Build history of the part. All positions in model axes, mm. Give positions to 0.01 mm unless a question says otherwise; leave off trailing zeros. Write each loop counter-clockwise with the first axis right and the second up, starting at its lowest first coordinate (ties: lowest second). Pieces come first, ordered by that corner, then holes. Notation, with made-up numbers: (32.25, 18) -> (61.25, 18) arc R26 ccw to (61.25, 40) -> close; hole circle Ø8 at (78.5, 16.5). An arc over 180 degrees is marked (long way). Write item = value, one per line. Start each with the question number.
Q1. Wall check: line 1 (Y direction, x = 0, z = 0.6); line 2 (X direction, y = 4.5, z = 1.4); line 3 (Y direction, x = -15, z = 0.9). Give the ranges that are in metal, low to high.
Q2. Saw through at B-B, the plane y = -18.5. List the corners of the cut face in (x, z).
Q3. Saw through at C-C, the plane y = 2.5. List the corners of the cut face in (x, z), then the cut area to 3 significant figures.
Q4. Drop flat-ended pins along their axis: P1, Ø1.9, axis at x = 15, y = 16.5, coming from the -Z side; P2, Ø10, axis at x = 13, y = 11.5, coming from the -Z side; P3, Ø1, axis at y = 6.5, z = 1.5, coming from the +X side. Give the stop position or say it passes through.
Q5. Saw through at D-D, the plane z = 1.05. Give the number of separate pieces and of enclosed holes in the cut face, then the cut area to 3 significant figures.
Q6. Saw through at A-A, the plane x = 0. List the corners of the cut face in (y, z).
Autodesk Inventor part; units mm, degrees
ref_plane "YZ Plane" through (0, 0, 0) normal (1, 0, 0) x (0, 1, 0)
ref_plane "XZ Plane" through (0, 0, 0) normal (0, 1, 0) x (-1, 0, 0)
ref_plane "XY Plane" through (0, 0, 0) normal (0, 0, 1) x (1, 0, 0)
sketch "スケッチ1" plane through (0, 0, 0) normal (0, 0, 1) x (1, 0, 0)
  circle A0 centre (0, 0) radius 11
  line L0 (-10, 22) -> (10, 22)
  line L1 (17.75, -44.5) -> (-17.75, -44.5)
  line L2 (-15, 16.5) -> (15, 16.5) construction
  line L3 (15, 16.5) -> (15, -42) construction
  line L4 (15, -42) -> (-15, -42) construction
  line L5 (-15, -42) -> (-15, 16.5) construction
  circle A1 centre (-15, 16.5) radius 1.55
  circle A2 centre (15, 16.5) radius 1.55
  circle A3 centre (-15, -42) radius 1.55
  circle A4 centre (15, -42) radius 1.55
  line L6 (-17.75, -44.5) -> (-20, -44.5)
  line L7 (-20, -44.5) -> (-20, 17.12)
  line L8 (-10, 22) -> (-20, 17.12)
  line L9 (0, 22) -> (0, -44.5) construction
  line L10 (-20, -23) -> (-22, -23)
  line L11 (-22, -23) -> (-22, -13)
  line L12 (-22, -13) -> (-20, -13)
  line L13 (17.75, -44.5) -> (20, -44.5)
  line L14 (20, -44.5) -> (20, 17.12)
  line L15 (10, 22) -> (20, 17.12)
  line L16 (20, -23) -> (22, -23)
  line L17 (22, -23) -> (22, -13)
  line L18 (22, -13) -> (20, -13)
  line L19 (13.5, -1) -> (-13.5, -1) construction
  line L20 (-13.5, -1) -> (-13.5, -28) construction
  line L21 (-13.5, -28) -> (13.5, -28) construction
  line L22 (13.5, -28) -> (13.5, -1) construction
  circle A5 centre (-13.5, -1) radius 1.35
  circle A6 centre (-13.5, -28) radius 1.35
  circle A7 centre (13.5, -1) radius 1.35
  circle A8 centre (13.5, -28) radius 1.35
  line L23 (10.01, -42) -> (-10.01, -42)
  line L24 (-10.01, -42) -> (-10.01, -39.48)
  line L25 (-10.01, -39.48) -> (10.01, -39.48)
  line L26 (10.01, -39.48) -> (10.01, -42)
  circle A9 centre (-8.96, -39.48) radius 1.05
  circle A10 centre (-8.96, -42) radius 1.05
  circle A11 centre (8.96, -42) radius 1.05
  circle A12 centre (8.96, -39.48) radius 1.05
  line L27 (-10.1, 19.01) -> (10.1, 19.01)
  line L28 (10.1, 19.01) -> (10.1, 16.49)
  line L29 (10.1, 16.49) -> (-10.1, 16.49)
  line L30 (-10.1, 16.49) -> (-10.1, 19.01)
  circle A13 centre (-9.05, 19.01) radius 1.05
  circle A14 centre (-9.05, 16.49) radius 1.05
  circle A15 centre (9.05, 16.49) radius 1.05
  circle A16 centre (9.05, 19.01) radius 1.05
  arc A17 (-20, -25.1) -> (-20, -23) centre (-20, -24.05) ccw
  arc A18 (-20, -13) -> (-20, -10.9) centre (-20, -11.95) ccw
  arc A19 (20, -23) -> (20, -25.1) centre (20, -24.05) ccw
  arc A20 (20, -10.9) -> (20, -13) centre (20, -11.95) ccw
  point P0 (7.91, -42)
  point P1 (-7.91, -42)
  point P2 (-7.91, -39.48)
  point P3 (7.91, -39.48)
  point P4 (8, 16.49)
  point P5 (-8, 16.49)
  point P6 (-10.1, 19.01)
  point P7 (-8, 19.01)
  point P8 (8, 19.01)
  point P9 (0, -39.48)
  point P10 (0, 16.49)
  point P11 (0, 19.01)
  point P12 (20, -25.1)
  dimension "d111" = 2.1
  dimension "d140" = 2.1
  dimension "d141" = 2.1
  dimension "d147" = 2.1
  dimension "d0" = 22
  dimension "d1" = 20
  dimension "d3" = 35.5
  dimension "d6" = 44.5
  dimension "d12" = 66.5
  dimension "d21" = 58.5
  dimension "d23" = 5.5
  dimension "d25" = 3.1
  dimension "d26" = 3.1
  dimension "d27" = 3.1
  dimension "d28" = 3.1
  dimension "d38" = 2
  dimension "d39" = 10
  dimension "d42" = 15
  dimension "d43" = 30
  dimension "d44" = 35
  dimension "d45" = 15
  dimension "d62" = 27
  dimension "d63" = 27
  dimension "d64" = 13.5
  dimension "d65" = 1
  dimension "d66" = 2.7
  dimension "d67" = 2.7
  dimension "d68" = 2.7
  dimension "d69" = 2.7
  dimension "d104" = 20.02
  dimension "d105" = 2.52
  dimension "d109" = 2.1
  dimension "d110" = 2.1
  dimension "d112" = 2.1
  dimension "d129" = 16.5
  dimension "d131" = 39.48
  dimension "d133" = 2.52
  dimension "d134" = 20.2
  dimension "d136" = 5.51
  dimension "d139" = 2.1
  dimension "d149" = 40
  dimension "d150" = 2.75
  dimension "d151" = 1.05
  dimension "d152" = 1.05
extrude "押し出し1" add sketch "スケッチ1" along normal blind 2 contours L0 L15 L14 A20 A19 L13 L1 L6 L7 A17 A18 L8 | L7 L10 L11 L12 | L18 L17 L16 L14
sketch "スケッチ2" plane through (0, 0, 2) normal (0, 0, 1) x (1, 0, 0)
  circle A0 centre (-13.5, -28) radius 1.35
  circle A1 centre (13.5, -28) radius 1.35
  circle A2 centre (-13.5, -1) radius 1.35
  circle A3 centre (13.5, -1) radius 1.35
  circle A4 centre (0, 0) radius 13 construction
  line L0 (20, -44.5) -> (20, 17.12)
  line L1 (-20, 17.12) -> (-20, -44.5)
  line L2 (10, 22) -> (-10, 22)
  line L3 (0, 22) -> (0, -44.5) construction
  line L4 (-20, -44.5) -> (20, -44.5)
  circle A5 centre (-13.5, -1) radius 2.6 construction
  circle A6 centre (13.5, -1) radius 2.6 construction
  circle A7 centre (-13.5, -28) radius 2.6 construction
  circle A8 centre (13.5, -28) radius 2.6 construction
  arc A9 (-3.8182, 12.4266) -> (-12.8912, 1.6787) centre (0, 0) ccw
  arc A10 (12.8912, 1.6787) -> (3.8182, 12.4266) centre (0, 0) ccw
  arc A11 (-12.4916, -3.6) -> (12.4916, -3.6) centre (0, 0) ccw
  arc A12 (-10.9, -28) -> (-13.5, -25.4) centre (-13.5, -28) ccw
  arc A13 (13.5, -25.4) -> (10.9, -28) centre (13.5, -28) ccw
  line L5 (-10.9, -28) -> (10.9, -28)
  line L6 (-13.4907, -30.6) -> (13.5093, -30.6)
  arc A14 (-7.91, -39.48) -> (-10.01, -39.48) centre (-8.96, -39.48) ccw
  circle A15 centre (-8.96, -39.48) radius 2.45 construction
  arc A16 (10.01, -39.48) -> (7.91, -39.48) centre (8.96, -39.48) ccw
  circle A17 centre (8.96, -39.48) radius 2.45 construction
  line L7 (-13.4907, -30.6) -> (-13.4907, -37.03)
  line L8 (-13.4907, -37.03) -> (13.5093, -37.03)
  line L9 (13.5093, -37.03) -> (13.5093, -30.6)
  line L10 (-17.5, 12.5022) -> (-3.8182, 12.4266)
  line L11 (-17.5, 12.5022) -> (-17.5, 1.6787)
  line L12 (-17.5, 1.6787) -> (-12.8912, 1.6787)
  arc A18 (12.8912, 1.6787) -> (3.8182, 12.4266) centre (0, 0) ccw
  line L13 (17.5, 12.5022) -> (3.8182, 12.4266)
  line L14 (17.5, 12.5022) -> (17.5, 1.6787)
  line L15 (17.5, 1.6787) -> (12.8912, 1.6787)
  line L16 (-17.48, -3.6) -> (-12.4916, -3.6)
  line L17 (-17.48, -3.6) -> (-17.48, -25.4)
  line L18 (-17.48, -25.4) -> (-13.5, -25.4)
  line L19 (17.5, -3.6) -> (12.4916, -3.6)
  line L20 (17.5, -3.6) -> (17.5, -25.4)
  line L21 (17.5, -25.4) -> (13.5, -25.4)
  dimension "d76" = 26
  dimension "d82" = 5.2
  dimension "d83" = 5.2
  dimension "d84" = 5.2
  dimension "d85" = 5.2
  dimension "d88" = 23.8182
  dimension "d89" = 32.8912
  dimension "d92" = 21.8
  dimension "d94" = 13
  dimension "d115" = 4.9
  dimension "d116" = 4.9
  dimension "d117" = 6.5093
  dimension "d118" = 7.47
  dimension "d123" = 10.8236
  dimension "d124" = 2.5
  dimension "d125" = 21.8
  dimension "d126" = 34.98
  dimension "d127" = 2.5
extrude "押し出し2" cut sketch "スケッチ2" against normal blind 2 contours A9 L12 L11 L10 | A10 L13 L14 L15 | A11 L19 L20 L21 A13 L5 A12 L18 L17 L16 | L6 L9 L8 L7
fillet "フィレット2" radius 2 20 edges at (-17.5, 12.5022, 1) (-3.8182, 12.4266, 1) (17.5, 12.5022, 1) (-12.8912, 1.6787, 1) (17.5, 1.6787, 1) (3.8182, 12.4266, 1) (-17.5, 1.6787, 1) (12.8912, 1.6787, 1) (17.5, -3.6, 1) (12.4916, -3.6, 1) (-12.4916, -3.6, 1) (-17.48, -3.6, 1) (-17.48, -25.4, 1) (-10.9, -28, 1) (17.5, -25.4, 1) (10.9, -28, 1) (13.5093, -37.03, 1) (-13.4907, -37.03, 1) (-13.4907, -30.6, 1) (13.5093, -30.6, 1)
fillet "フィレット3" radius 1 6 edges at (-20, -44.5, 1) (20, -44.5, 1) (-20, 17.12, 1) (-10, 22, 1) (10, 22, 1) (20, 17.12, 1)
equation "\"d26\" = d25"
equation "\"d27\" = d25"
equation "\"d28\" = d25"
equation "\"d67\" = d66"
equation "\"d68\" = d66"
equation "\"d69\" = d66"
properties part number "胴体_サブフレーム_仮１"
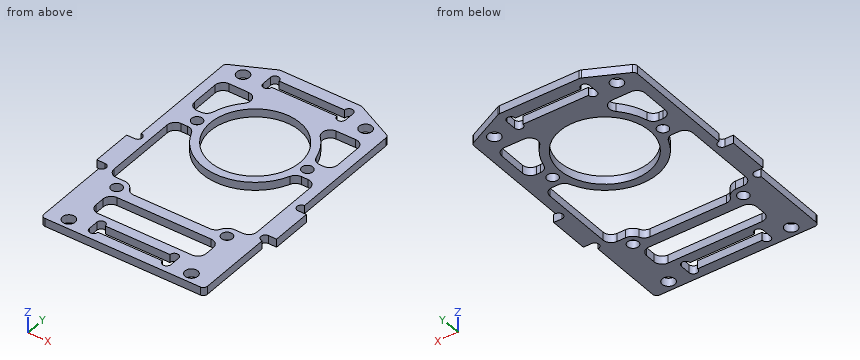
Report:
q1.line_1 = -44.5 to -42, -39.48 to -37.03, -30.6 to -28, -13 to -11, 11 to 16.49, 19.01 to 22
q1.line_2 = -20 to -17.5, -12.2 to -10.04, 10.04 to 12.2, 17.5 to 20
q1.line_3 = -44.5 to -43.55, -40.45 to -25.4, -3.6 to 1.68, 12.49 to 14.95, 18.05 to 19.56
q2.outline = (-22, 0) -> (-17.48, 0) -> (-17.48, 2) -> (-22, 2) -> close; (17.5, 0) -> (22, 0) -> (22, 2) -> (17.5, 2) -> close
q3.outline = (-20, 0) -> (-17.12, 0) -> (-17.12, 2) -> (-20, 2) -> close; (-12.93, 0) -> (-10.71, 0) -> (-10.71, 2) -> (-12.93, 2) -> close; (10.71, 0) -> (12.93, 0) -> (12.93, 2) -> (10.71, 2) -> close; (17.12, 0) -> (20, 0) -> (20, 2) -> (17.12, 2) -> close
q3.area = 20.4 mm2
q4.P1 = through
q4.P2 = 0
q4.P3 = 20
q5.separate_pieces = 1
q5.enclosed_holes = 15
q5.area = 1,140 mm2
q6.outline = (-44.5, 0) -> (-42, 0) -> (-42, 2) -> (-44.5, 2) -> close; (-39.48, 0) -> (-37.03, 0) -> (-37.03, 2) -> (-39.48, 2) -> close; (-30.6, 0) -> (-28, 0) -> (-28, 2) -> (-30.6, 2) -> close; (-13, 0) -> (-11, 0) -> (-11, 2) -> (-13, 2) -> close; (11, 0) -> (16.49, 0) -> (16.49, 2) -> (11, 2) -> close; (19.01, 0) -> (22, 0) -> (22, 2) -> (19.01, 2) -> close
